Geometry: final body of the model. Coordinates: model frame, mm. Give positions to 0.01 mm unless a question says otherwise; leave off trailing zeros. Write each loop counter-clockwise with the first axis right and the second up, starting at its lowest first coordinate (ties: lowest second). Pieces come first, ordered by that corner, then holes. Notation, with made-up numbers: (39.25, -1) -> (43.25, -1) arc R26 cw to (43.25, 14) -> close; hole circle Ø10 at (67, 33). An arc over 180 degrees is marked (long way). Answer in a Markdown table with one row per item. Add a question column.
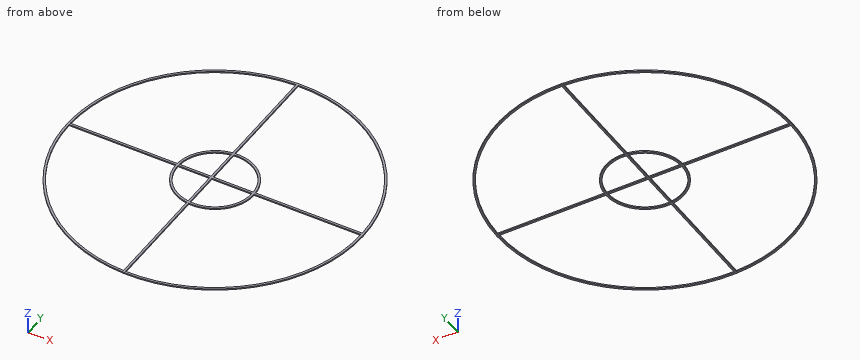
from build123d import *

# Parameters (mm, degrees)
F0_R     = 70
F1_DEPTH = 0.6


with BuildPart() as f1:
    # F0 (on Top) → F1 (new body)
    with BuildSketch(Plane.XY):
        with Locations((0.124242, -0.496998)):
            Circle(F0_R)
        with BuildLine():
            ThreePointArc((-2.352914, -69.452517), (-49.534211, -48.403554), (-68.875758, -0.496998))
            Line((-68.875758, -0.496998), (-18.375758, -0.496998))
            ThreePointArc((-18.375758, -0.496998), (-13.805536, -12.671204), (-2.352914, -18.830401))
            Line((-2.352914, -18.830401), (-2.352914, -69.452517))
        make_face(mode=Mode.SUBTRACT)
        with BuildLine():
            ThreePointArc((-2.352914, -17.820788), (-13.096958, -11.962157), (-17.375758, -0.496998))
            Line((-17.375758, -0.496998), (-2.352914, -0.496998))
            Line((-2.352914, -0.496998), (-2.352914, -17.820788))
        make_face(mode=Mode.SUBTRACT)
        with BuildLine():
            ThreePointArc((69.124242, -0.496998), (48.389531, -49.806853), (-1.352914, -69.481184))
            Line((-1.352914, -69.481184), (-1.352914, -18.937931))
            ThreePointArc((-1.352914, -18.937931), (12.6726, -14.090698), (18.624242, -0.496998))
            Line((18.624242, -0.496998), (69.124242, -0.496998))
        make_face(mode=Mode.SUBTRACT)
        with BuildLine():
            Line((-1.352914, -17.934544), (-1.352914, -0.496998))
            Line((-1.352914, -0.496998), (17.624242, -0.496998))
            ThreePointArc((17.624242, -0.496998), (11.964845, -13.383041), (-1.352914, -17.934544))
        make_face(mode=Mode.SUBTRACT)
        with BuildLine():
            ThreePointArc((-68.868512, 0.503002), (-49.185749, 47.768154), (-2.352914, 68.458522))
            Line((-2.352914, 68.458522), (-2.352914, 17.836406))
            ThreePointArc((-2.352914, 17.836406), (-13.47129, 12.049377), (-18.348712, 0.503002))
            Line((-18.348712, 0.503002), (-68.868512, 0.503002))
        make_face(mode=Mode.SUBTRACT)
        with BuildLine():
            Line((-2.352914, 16.826792), (-2.352914, 0.503002))
            Line((-2.352914, 0.503002), (-17.347164, 0.503002))
            ThreePointArc((-17.347164, 0.503002), (-12.763846, 11.34138), (-2.352914, 16.826792))
        make_face(mode=Mode.SUBTRACT)
        with BuildLine():
            Line((17.595647, 0.503002), (-1.352914, 0.503002))
            Line((-1.352914, 0.503002), (-1.352914, 16.940548))
            ThreePointArc((-1.352914, 16.940548), (11.591684, 12.722222), (17.595647, 0.503002))
        make_face(mode=Mode.SUBTRACT)
        with BuildLine():
            ThreePointArc((-1.352914, 68.487189), (48.030936, 49.161321), (69.116995, 0.503002))
            Line((69.116995, 0.503002), (18.597195, 0.503002))
            ThreePointArc((18.597195, 0.503002), (12.300481, 13.431002), (-1.352914, 17.943935))
            Line((-1.352914, 17.943935), (-1.352914, 68.487189))
        make_face(mode=Mode.SUBTRACT)
    extrude(amount=F1_DEPTH)


solid = f1.part
Q1. Section B-B on y = -56. Return loops of the section in (x, z), and give its area (3 significant figures).
Q2. Section D-D on x = -56. Return loops of the section in (y, z).
Q3. Section A-A on x = -12.5. Return loops of the section in (y, z).
Q4. Line query: probe 1 along Y at (x, z) = (2.5, 0.45); probe 2 along Y at (x, z) = (39, 0.1); probe 3 along X at (y, z) = (24, 0.1). Output: solid intervals per line, ascending. Write a range as from..to.
Q5. Section C-C on z = 0.3. Count the separate pieces of the cut face and the enclosed holes in it, and give its area (3 significant figures).
Checks:
| question | item | result |
|---|---|---|
| 1 | outline | (-42.53, 0) -> (-40.87, 0) -> (-40.87, 0.6) -> (-42.53, 0.6) -> close; (-2.35, 0) -> (-1.35, 0) -> (-1.35, 0.6) -> (-2.35, 0.6) -> close; (41.12, 0) -> (42.78, 0) -> (42.78, 0.6) -> (41.12, 0.6) -> close |
| 1 | area | 2.59 mm^2 |
| 2 | outline | (-42.33, 0) -> (-40.64, 0) -> (-40.64, 0.6) -> (-42.33, 0.6) -> close; (-0.5, 0) -> (0.5, 0) -> (0.5, 0.6) -> (-0.5, 0.6) -> close; (39.64, 0) -> (41.34, 0) -> (41.34, 0.6) -> (39.64, 0.6) -> close |
| 3 | outline | (-69.35, 0) -> (-68.33, 0) -> (-68.33, 0.6) -> (-69.35, 0.6) -> close; (-14.02, 0) -> (-12.62, 0) -> (-12.62, 0.6) -> (-14.02, 0.6) -> close; (-0.5, 0) -> (0.5, 0) -> (0.5, 0.6) -> (-0.5, 0.6) -> close; (11.62, 0) -> (13.03, 0) -> (13.03, 0.6) -> (11.62, 0.6) -> close; (67.34, 0) -> (68.36, 0) -> (68.36, 0.6) -> (67.34, 0.6) -> close |
| 4 | probe 1 | -70.46..-69.46, -18.84..-17.83, -0.5..0.5, 16.84..17.85, 68.46..69.46 |
| 4 | probe 2 | -58.71..-57.5, -0.5..0.5, 56.51..57.72 |
| 4 | probe 3 | -65.45..-64.38, -2.35..-1.35, 64.63..65.7 |
| 5 | separate pieces | 1 |
| 5 | enclosed holes | 8 |
| 5 | area | 821 mm^2 |
